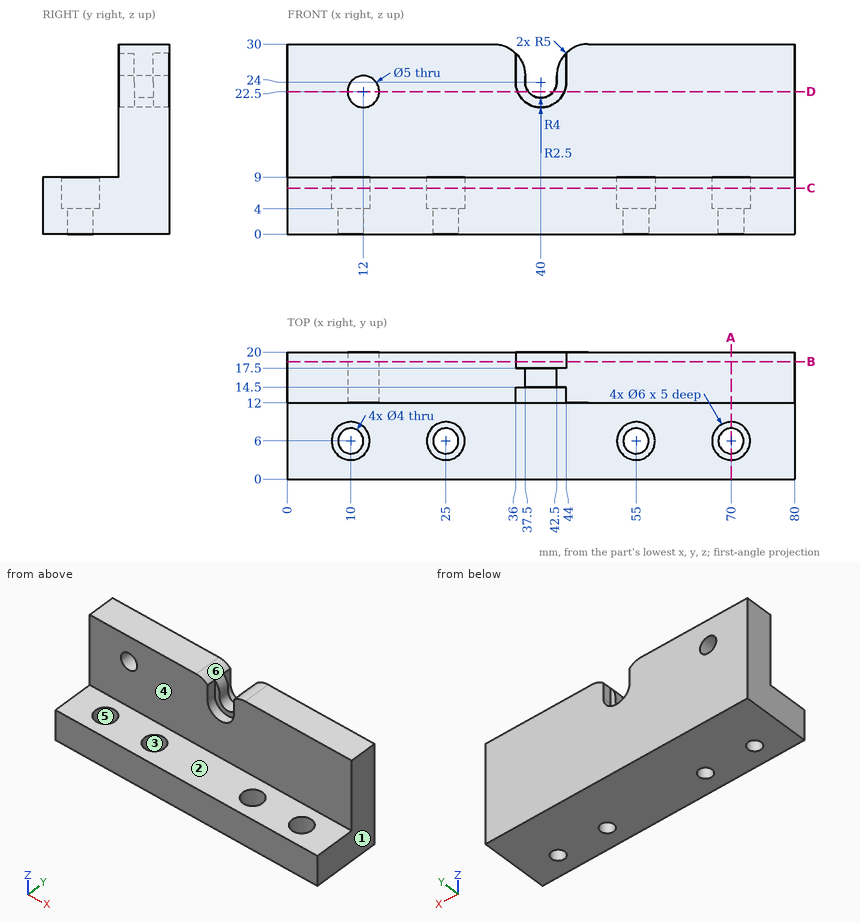
Geometry: see drawing. Coordinates: mm, zero at the bounding-box minimum. A direction names the side the tool comes from. Give positions to 0.01 mm unless a question says otherwise; leave off trailing zeros. Loops run counter-clockwise (first coordinate to the right, second up) from the corner with the lowest first, then second, coordinate; pieces in that order, holes last. Notation, with made-up numbers: M 75.25,83.25 L 97.25,83.25 A5 ccw 97.25,89.25 Z; hole C 20.5,84 d7. An arc over 180 degrees is marked long. Answer as CSV lines item,"result". Start each with the question number.
1. Pull-direction query (X, two-part tool) for the marked faces 1, 2 and 3; classes: released by +X, released by -X, zero draft, split by the parting line, or undercut.
2. Reachability of the marked faces 4, 5 and 6 from +Z, -Z, +X, -X, +Y, -Y: full face, straight path, thin tool, end or side. Return the list, or none.
3. Section A-A on x = 70. Return loops of the section in (y, z).
4. Section B-B on y = 18.5. Return loops of the section in (x, z).
5. Section C-C on z = 7.25. Return loops of the section in (x, y).
6. Pin query (flat end, axial travel): P1, Ø5, axis at x = 26, y = 6, coming from the +Z side; P2, Ø6.5, axis at x = 50.5, z = 20.5, coming from the -Y side; P3, Ø4, axis at x = 39, z = 26, coming from the +Y side. Return the tip coordinate at first contact, or that it passes through.
7. Section D-D on z = 22.5. Return loops of the section in (x, y).
8. Line query: L1, parallel to Y at x = 25, z = 7.4; L2, parallel to Z at x = 6.5, y = 4; L3, parallel to X at y = 14, z = 28.25. Output: solid intervals per line, ascending.
Computed values:
1,face 1,"released by +X"
1,face 2,"zero draft"
1,face 3,"undercut"
2,face 4,"+Z, +X, -X, -Y"
2,face 5,"+Z"
2,face 6,"+Z, +Y, -Y"
3,outline,"M 0,0 L 4,0 L 4,4 L 3,4 L 3,9 L 0,9 Z; M 8,0 L 20,0 L 20,30 L 12,30 L 12,9 L 9,9 L 9,4 L 8,4 Z"
4,outline,"M 0,0 L 80,0 L 80,30 L 47.5,30 A5 ccw 44,28.57 L 44,24 A4 cw 36,24 L 36,28.57 A5 ccw 32.5,30 L 0,30 Z; hole C 12,22.5 d5"
5,outline,"M 0,0 L 80,0 L 80,20 L 0,20 Z; hole C 10,6 d6; hole C 25,6 d6; hole C 55,6 d6; hole C 70,6 d6"
6,P1,"stops at z = 9"
6,P2,"stops at y = 12"
6,P3,"stops at y = 17.5"
7,outline,"M 0,12 L 9.5,12 L 9.5,20 L 0,20 Z; M 14.5,12 L 36.29,12 L 36.29,14.5 L 38,14.5 L 38,17.5 L 36.29,17.5 L 36.29,20 L 14.5,20 Z; M 42,14.5 L 43.71,14.5 L 43.71,12 L 80,12 L 80,20 L 43.71,20 L 43.71,17.5 L 42,17.5 Z"
8,L1,"y = 0 to 3, 9 to 20"
8,L2,"z = 0 to 9"
8,L3,"x = 0 to 36, 44 to 80"
